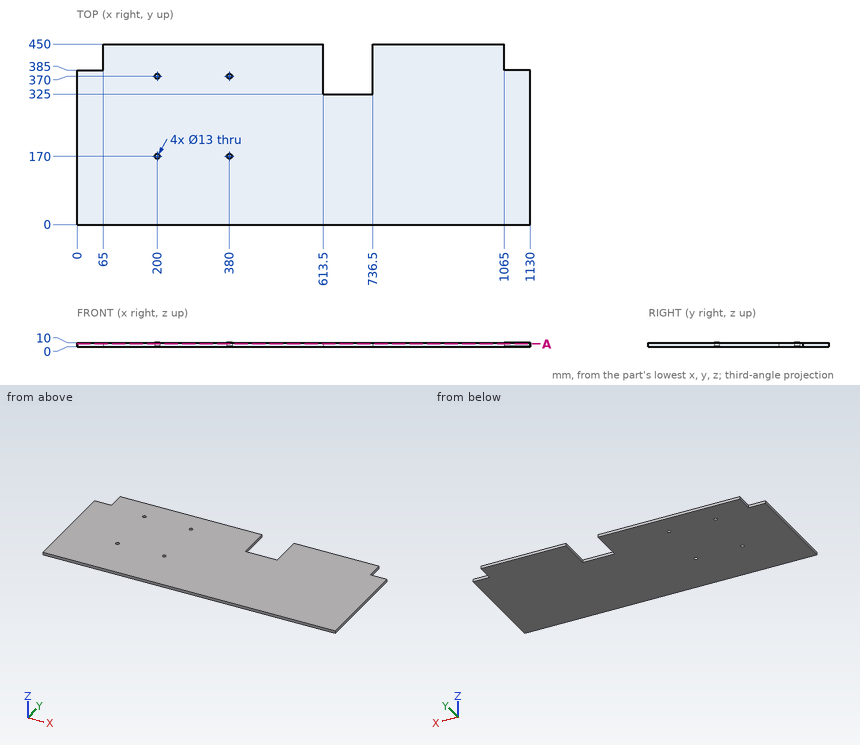
Study the drawing (mm; zero at the part's minimum x, y, z) and answer. Coordinates: 2 decimals unless noted, no trailing zeros. Write each loop counter-clockwise with the first axis right and the second up, starting at its lowest first coordinate (ties: lowest second). Pieces come first, ordered by that corner, then holes. Notation, with made-up numbers: (68.5, 59.25) - (118.5, 59.25) arc R26 ccw to (118.5, 96.25) - close; hole circle Ø8 at (-14, -36). An arc over 180 degrees is marked (long way). One line per item, written item: value.
1) Each of these flat-tipped pins is pushed along its axis until it touches: pin 1 Ø3 at (y, z) = (362.5, 5.5) entering from -X; pin 2 Ø3 at (x, z) = (651, 7) entering from +Y; pin 3 Ø3 at (y, z) = (393, 3.5) entering from +X. Where does it stop, or does it pass through?
Geometry check:
pin 1: stops at x = 0
pin 2: stops at y = 325
pin 3: stops at x = 1065
2) Find section A-A (z = 6.5). Give the vertices of the cut face in (x, y), and give its area (3 significant figures).
Geometry check:
outline: (0, 0) - (1130, 0) - (1130, 385) - (1065, 385) - (1065, 450) - (736.5, 450) - (736.5, 325) - (613.5, 325) - (613.5, 450) - (65, 450) - (65, 385) - (0, 385) - close; hole circle Ø13 at (200, 170); hole circle Ø13 at (200, 370); hole circle Ø13 at (380, 170); hole circle Ø13 at (380, 370)
area: 484,000 mm2
3) Consider line 1 along X through (y, z) = (370, 2.5); line 2 along Y through (x, z) = (200, 3); line 3 along X through (y, z) = (359, 2). Determine where each line is inside the solid, lowest interval first. Write a range as from..to.
Geometry check:
line 1: x = 0..193.5, 206.5..373.5, 386.5..613.5, 736.5..1130
line 2: y = 0..163.5, 176.5..363.5, 376.5..450
line 3: x = 0..613.5, 736.5..1130
